The listing builds one solid part. Answer for the finished solid, in the listing's coordinates (mm). A direction names the side the tool comes from. Round coordinates to 2 decimals unless told otherwise and drop trailing zeros. Order: outer loops, then holes, each group sorted by start corner. A loop starts at its lowest first (then second) coordinate and runs counter-clockwise, first axis right, second up. Notation, with made-up numbers: (14, 9.5) -> (71, 9.5) arc R25 cw to (71, 39.5) -> close; hole circle Ø5 at (57.25, 62). An arc over 180 degrees is marked (long way). Return JSON: item names as keys, results as strings. Group by question number.
(1) Which of the six approach directions +Z, -Z, +X, -X, +Y, -Y give full straight-line access (tool end or side, diameter ignored) to faces 1 (the face through (39.14, 39.1, 1.52)), 2 (the face through (20, 20, 3))?
(2) Consider line 1 (Z direction, x = 21, y = 38.5); line 2 (Y direction, x = 23, z = 17.5); line 3 (X direction, y = 15.5, z = 18.5). Determine where each line is inside the solid, lowest interval first. Write a range as [from, to].
(3) The part is cut by section C-C (z = 29.5). Determine the outline of the cut face in (x, y), plus the area to 3 significant figures.
(4) Each of these flat-tipped pins is pushed along its axis until it touches: pin 1 (1 mm diameter, centred on x = 4.5, y = 8.5, fed in from +Z); pin 2 (1.5 mm diameter, centred on y = 28, z = 27, fed in from -X); pin 3 (4 mm diameter, centred on y = 14.5, z = 16.5, fed in from +X). Where does it stop, or does it pass through?
(5) The part is cut by section D-D (z = 15). Determine the outline of the cut face in (x, y), plus the area to 3 significant figures.
(6) Determine the mould class of faces 3 (the face through (11, 34, 3)), 4 (the face through (40, 20, 1)), 5 (the face through (18.356, 12.598, 27.724)) for opening direction X: +X half, -X half, draft (parallel to the pull), parting line (faces both ways), or undercut.
(7) The part is cut by section A-A (x = 20). Determine the outline of the cut face in (y, z), plus the area to 3 significant figures.
from build123d import *

# Parameters (mm, degrees)
BOX_W     = 40
BOX_H     = 40
BOX_DEPTH = 3
FILLET_R  = 3


with BuildPart() as cone001:
    # Cone001 → Cone001 (revolve)
    with BuildSketch(Plane(origin=(20, 20, 3), x_dir=(1, 0, 0), z_dir=(0, -1, 0))):
        Polygon((0, 0), (15, 0), (3, 40), (0, 40), align=None)
    revolve(axis=Axis((20, 20, 3), (0, 0, 1)))


with BuildPart() as cut:
    # Cone → Cone (revolve)
    with BuildSketch(Plane(origin=(20, 20, 3), x_dir=(1, 0, 0), z_dir=(0, -1, 0))):
        Polygon((0, 0), (16, 0), (4, 40), (0, 40), align=None)
    revolve(axis=Axis((20, 20, 3), (0, 0, 1)))

    # Cut: cut Cone001
    add(cone001.part, mode=Mode.SUBTRACT)


with BuildPart() as obj1:
    # Box → Box (new body)
    with BuildSketch(Plane.XY):
        with Locations((20, 20)):
            Rectangle(BOX_W, BOX_H)
    extrude(amount=BOX_DEPTH)

    # Fillet
    fillet_edges = [obj1.edges().sort_by_distance(p)[0] for p in [
        (0, 0, 1.5),
        (0, 40, 1.5),
        (40, 0, 1.5),
        (40, 40, 1.5),
    ]]
    fillet(fillet_edges, radius=FILLET_R)

    # Fusion: union Cut
    add(cut.part)


solid = obj1.part
Answer below:
{
 "1": {"face 1": "+Z, -Z, +X, +Y", "face 2": "none"},
 "2": {"line 1": "z = [0, 3]", "line 2": "y = [8.74, 9.78], [30.22, 31.26]", "line 3": "x = [9.58, 10.68], [29.32, 30.42]"},
 "3": {"outline": "circle Ø16.1 at (20, 20); hole circle Ø14.1 at (20, 20)", "area": "47.4 mm²"},
 "4": {"pin 1": "stops at z = 3", "pin 2": "stops at x = 14.94", "pin 3": "stops at x = 31.68"},
 "5": {"outline": "circle Ø24.8 at (20, 20); hole circle Ø22.8 at (20, 20)", "area": "74.8 mm²"},
 "6": {"face 3": "draft", "face 4": "+X half", "face 5": "undercut"},
 "7": {"outline": "(0, 0) -> (40, 0) -> (40, 3) -> (36, 3) -> (24, 43) -> (23, 43) -> (35, 3) -> (5, 3) -> (17, 43) -> (16, 43) -> (4, 3) -> (0, 3) -> close", "area": "200 mm²"}
}
